Input: part model. Units: mm. Frame: model coordinates. Coordinates: 2 decimals unless noted, no trailing zeros. Loops run counter-clockwise (first coordinate to the right, second up) from the corner with the lowest first, then second, coordinate; pieces in that order, holes last.
Item 1: Section A-A on x = 0. Return loops of the section in (y, z).
Item 2: Ray query, line 1 along Y through (x, z) = (0, 0.4); line 2 along X through (y, z) = (38, 0.5); line 3 along X through (y, z) = (9, 1.05). Return the intervals inside material, ascending.
Item 3: Section B-B on y = 38. Return loops of the section in (x, z), and give its area (3 significant figures).
Autodesk Inventor part; units mm, degrees
ref_plane "YZ Plane" through (0, 0, 0) normal (1, 0, 0) x (0, 1, 0)
ref_plane "XZ Plane" through (0, 0, 0) normal (0, 1, 0) x (-1, 0, 0)
ref_plane "XY Plane" through (0, 0, 0) normal (0, 0, 1) x (1, 0, 0)
sketch "Sketch1" plane through (0, 0, 0) normal (0, 0, 1) x (1, 0, 0)
  line L0 (-54, -40.5) -> (54, -40.5)
  line L1 (54, -40.5) -> (54, 40.5)
  line L2 (54, 40.5) -> (-54, 40.5)
  line L3 (-54, 40.5) -> (-54, -40.5)
  point P0 (0, 0)
  dimension "d0" = 108
  dimension "d1" = 81
  dimension "d2" = 40.5
  dimension "d3" = 54
extrude "Extrusion1" add sketch "Sketch1" along normal blind 1.5875
hole "Hole2" at (50, -38, 1.5875) direction (0, 0, -1) diameter 2.6924 end through all
mirror "Mirror1" about plane through (0, 0, 0) normal (0, 1, 0) of "Hole2"
hole "Hole3" [suppressed]
hole "Hole4" [suppressed]
mirror "Mirror2" about plane through (0, 0, 0) normal (1, 0, 0) of "Hole2", "Mirror1"
hole "Hole5" at (0, -38, 1.5875) direction (0, 0, -1) diameter 2.6924 end through all
mirror "Mirror3" about plane through (0, 0, 0) normal (0, 1, 0) of "Hole5"
hole "Hole6" at (51.25, 0, 0) direction (0, 0, 1) diameter 2.6924 end through all
mirror "Mirror4" about plane through (0, 0, 0) normal (1, 0, 0) of "Hole6"
hole "Hole_spring" at (-47.6, 17.5, 1.5875) direction (0, 0, -1) diameter 0.5 end through all
sketch "Sketch3" plane through (0, 0, 1.5875) normal (0, 0, 1) x (1, 0, 0)
  line L0 (-54, -40.5) -> (-54, 40.5)
  line L1 (-54, 40.5) -> (54, 40.5)
  line L2 (-47.6, 9.8024) -> (-47.6, -15.4623) construction
  circle A0 centre (-45.6, 3.5) radius 0.25
  circle A1 centre (-49.6, -10.0207) radius 0.25
  point P0 (0, 0)
  point P1 (-46.1616, -3.6859)
  dimension "d243" = 6.4
  dimension "d244" = 2
  dimension "d245" = 2
  dimension "d246" = 14.1
  dimension "d247" = 0.5
  dimension "d248" = 37
extrude "Holes_resistor" cut sketch "Sketch3" against normal through all
hole "Hole_via" at (-50, 9, 1.5875) direction (0, 0, -1) diameter 0.5 end through all
hole "Hole_spring_2" at (47.6, -17.5, 1.5875) direction (0, 0, -1) diameter 0.5 end through all
sketch "Sketch5" plane through (0, 0, 1.5875) normal (0, 0, 1) x (1, 0, 0)
  line L0 (54, -40.5) -> (-54, -40.5)
  line L1 (54, 40.5) -> (54, -40.5)
  line L2 (47.6, -11.3866) -> (47.6, 14.8402) construction
  circle A0 centre (49.6, 10.0207) radius 0.25
  circle A1 centre (45.6, -3.5) radius 0.25
  point P0 (0, 0)
  dimension "d271" = 6.4
  dimension "d272" = 2
  dimension "d273" = 2
  dimension "d274" = 0.5
  dimension "d275" = 14.1
  dimension "d276" = 37
extrude "Holes_resistor2" cut sketch "Sketch5" against normal through all
hole "Hole_via2" at (50, -9, 1.5875) direction (0, 0, -1) diameter 0.5 end through all
hole "Hole26" at (-52.5, 10.25, 1.5875) direction (0, 0, -1) diameter 0.6 end through all
hole "Hole27" at (52.5, -10.25, 1.5875) direction (0, 0, -1) diameter 0.6 end through all
sketch "Sketch8" plane through (0, 0, 1.5875) normal (0, 0, 1) x (1, 0, 0)
  line L0 (-54, -40.5) -> (-54, 40.5)
  line L1 (54, -40.5) -> (-54, -40.5)
  line L2 (54, 40.5) -> (54, -40.5)
  line L3 (-54, 40.5) -> (54, 40.5)
  line L4 (54.0603, -40.4195) -> (-54, -40.5) construction
  line L5 (-54, -40.5) -> (-54.0603, 40.4195) construction
  line L6 (-54.0603, 40.4195) -> (54, 40.5) construction
  line L7 (54, 40.5) -> (54.0603, -40.4195) construction
  point P0 (0, 0)
decal "Decal3"
sketch "Sketch9" plane through (0, 0, 0) normal (0, 0, -1) x (-1, 0, 0)
  line L0 (54, -40.5) -> (-54, -40.5)
  line L1 (54, 40.5) -> (54, -40.5)
  line L2 (-54, 40.5) -> (54, 40.5)
  line L3 (-54, -40.5) -> (-54, 40.5)
  line L4 (54.0603, -40.4195) -> (-54, -40.5) construction
  line L5 (-54, -40.5) -> (-54.0603, 40.4195) construction
  line L6 (-54.0603, 40.4195) -> (54, 40.5) construction
  line L7 (54, 40.5) -> (54.0603, -40.4195) construction
  point P0 (0, 0)
decal "Decal4"
equation "\"d283\" = d253"
properties part number "FOX-ME-127-05" material "FR4"
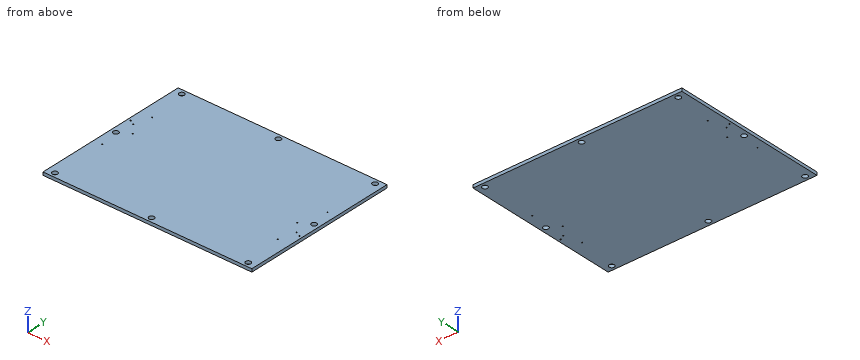
Results found:
1. outline: (-40.5, 0) - (-39.35, 0) - (-39.35, 1.59) - (-40.5, 1.59) - close; (-36.65, 0) - (36.65, 0) - (36.65, 1.59) - (-36.65, 1.59) - close; (39.35, 0) - (40.5, 0) - (40.5, 1.59) - (39.35, 1.59) - close
2. line 1: y = -40.5 to -39.35, -36.65 to 36.65, 39.35 to 40.5
2. line 2: x = -54 to -51.35, -48.65 to -1.35, 1.35 to 48.65, 51.35 to 54
2. line 3: x = -54 to -50.25, -49.75 to 54
3. outline: (-54, 0) - (-51.35, 0) - (-51.35, 1.59) - (-54, 1.59) - close; (-48.65, 0) - (-1.35, 0) - (-1.35, 1.59) - (-48.65, 1.59) - close; (1.35, 0) - (48.65, 0) - (48.65, 1.59) - (1.35, 1.59) - close; (51.35, 0) - (54, 0) - (54, 1.59) - (51.35, 1.59) - close
3. area: 159 mm2
